from build123d import *

# Parameters (mm, degrees)
SKETCH1_W           = 185
SKETCH1_H           = 100
BOSS_EXTRUDE1_DEPTH = 4
BOSS_EXTRUDE2_DEPTH = 4
SKETCH3_W           = 10
SKETCH3_H           = 100
BOSS_EXTRUDE3_DEPTH = 15
SKETCH4_W           = 20
SKETCH4_H           = 70
BOSS_EXTRUDE4_DEPTH = 6
SKETCH5_W           = 15
SKETCH5_H           = 20
BOSS_EXTRUDE5_DEPTH = 10
SKETCH6_R           = 4
BOSS_EXTRUDE6_DEPTH = 10


with BuildPart() as part:
    # Sketch1 → Boss-Extrude1 (new body)
    with BuildSketch(Plane(origin=(0, 0, 0), x_dir=(1, 0, 0), z_dir=(0, 1, 0))):
        with Locations((92.5, 50)):
            Rectangle(SKETCH1_W, SKETCH1_H)
    extrude(amount=BOSS_EXTRUDE1_DEPTH)

    # Sketch2 → Boss-Extrude2 (add)
    with BuildSketch(Plane(origin=(0, 4, 0), x_dir=(-1, 0, 0), z_dir=(0, 1, 0))):
        Polygon((-40, -115), (-40, -110), (0, -110), (0, -100), (-140, -100), (-140, -110), (-125, -110), (-125, -115), align=None)
    extrude(amount=-BOSS_EXTRUDE2_DEPTH)

    # Sketch3 → Boss-Extrude3 (add)
    with BuildSketch(Plane.XZ):
        with Locations((-3.300721775, -60)):
            Rectangle(SKETCH3_W, SKETCH3_H)
    extrude(amount=BOSS_EXTRUDE3_DEPTH)

    # Sketch4 → Boss-Extrude4 (add)
    with BuildSketch(Plane.XZ):
        with Locations((137.629312938, -55)):
            Rectangle(SKETCH4_W, SKETCH4_H)
    extrude(amount=BOSS_EXTRUDE4_DEPTH)

    # Sketch5 → Boss-Extrude5 (add)
    with BuildSketch(Plane.XZ):
        with Locations((162.5, -10)):
            Rectangle(SKETCH5_W, SKETCH5_H)
    extrude(amount=BOSS_EXTRUDE5_DEPTH)

    # Sketch6 → Boss-Extrude6 (add)
    with BuildSketch(Plane.XZ):
        with Locations(Location((180, -30, 0), (0, 0, 270))):
            Circle(SKETCH6_R)
        with Locations(Location((180, -90, 0), (0, 0, 270))):
            Circle(SKETCH6_R)
    extrude(amount=BOSS_EXTRUDE6_DEPTH)


solid = part.part
Design review of the part built by this model. Coordinates are the model's own, in mm. A direction names the side the tool comes from. Round coordinates to 2 decimals unless told otherwise and drop trailing zeros. Write each loop counter-clockwise with the first axis right and the second up, starting at its lowest first coordinate (ties: lowest second). Pieces come first, ordered by that corner, then holes. Notation, with made-up numbers: (80.5, 7.25) - (135.5, 7.25) arc R11 ccw to (135.5, 25.25) - close; hole circle Ø4 at (9, 17.5). An arc over 180 degrees is marked (long way). Return JSON: item names as keys, results as strings. Group by question number.
Item 1: Machinability: for faces 4 (the face through (162, 2, -100)), 5 (the face through (137, -3, -20)), 6 (the face through (162, -5, -20)), 7 (the face through (147.629, -3, -55)), 8 (the face through (180, -10, -30)), which of the approach directions +Z, -Z, +X, -X, +Y, -Y give a long, thin tool a straight path to every point of the face, cutting with its end or side? Answer none if there is none.
Item 2: We need section D-D on x = 25. Write out the cut boundary in (y, z).
Item 3: The part is to be moulded in two halves that separate along X. For faces 1 (the face through (170, -5, -10)), 2 (the face through (183.966, -4.93, -29.479)), 3 (the face through (-3, -15, -59)), say which applies: pulls with the +X half, pulls with the -X half, needs draft (parallel to the pull), parting line crosses it, or undercut.
Item 4: We need section B-B on x = 180. Write out the cut boundary in (y, z), and give its area (3 significant figures).
Item 5: Insertion check: P1, Ø5, axis at y = -7, z = -8.5, coming from the +X side; P2, Ø6.5, axis at x = -6, z = -41.5, coming from the +Y side; P3, Ø10, axis at x = 145, y = -5.5, coming from the -Z side; P4, Ø3, axis at x = 40, y = 0.5, coming from the +Z side. Each pin has a flat end and moves straight along its axis. Give the tip position at first contact, or say it passes through.
Item 6: We need section A-A on z = -36. Write out the cut boundary in (x, y).
Item 7: For probe 1 along X at (y, z) = (-1.5, -24.5); probe 2 along X at (y, z) = (-2.25, -14); probe 3 along X at (y, z) = (-13, -48.5), list the stretches that pass through material, from the lowest coordinate up. Write a range as [from, to].
Item 8: We need section C-C on x = 130. Write out the cut boundary in (y, z).
Model answer:
{
 "1": {"face 4": "-Z, +X, +Y, -Y", "face 5": "+Z, -Y", "face 6": "-Z, +X, -Y", "face 7": "+Z, -Z, -Y", "face 8": "+Z, -Z, +X, -Y"},
 "2": {"outline": "(0, -110) - (4, -110) - (4, 0) - (0, 0) - close"},
 "3": {"face 1": "pulls with the +X half", "face 2": "undercut", "face 3": "needs draft"},
 "4": {"outline": "(-10, -94) - (0, -94) - (0, -100) - (4, -100) - (4, 0) - (0, 0) - (0, -26) - (-10, -26) - (-10, -34) - (0, -34) - (0, -86) - (-10, -86) - close", "area": "560 mm²"},
 "5": {"P1": "stops at x = 170", "P2": "stops at y = 0", "P3": "stops at z = -90", "P4": "stops at z = 0"},
 "6": {"outline": "(-8.3, -15) - (1.7, -15) - (1.7, 0) - (127.63, 0) - (127.63, -6) - (147.63, -6) - (147.63, 0) - (185, 0) - (185, 4) - (0, 4) - (0, 0) - (-8.3, 0) - close"},
 "7": {"probe 1": "x = [-8.3, 1.7], [127.63, 147.63]", "probe 2": "x = [-8.3, 1.7], [155, 170]", "probe 3": "x = [-8.3, 1.7]"},
 "8": {"outline": "(-6, -90) - (0, -90) - (0, -110) - (4, -110) - (4, 0) - (0, 0) - (0, -20) - (-6, -20) - close"}
}
